CAD build for the part. Positions are in the model's coordinates, mm. A direction names the side the tool comes from. Coordinates: 2 decimals unless noted, no trailing zeros. Write each loop counter-clockwise with the first axis right and the second up, starting at its lowest first coordinate (ties: lowest second). Pieces come first, ordered by that corner, then holes. Notation, with made-up numbers: (65.25, 77) -> (98.25, 77) arc R28 cw to (98.25, 103) -> close; hole circle Ø3 at (31, -33). An arc over 180 degrees is marked (long way). Answer as CSV lines item,"result". Start each with the question number.
```python
from build123d import *

# Parameters (mm, degrees)
SKETCH1_R           = 12.5
BOSS_EXTRUDE1_DEPTH = 125
CUT_EXTRUDE1_START  = -20
CUT_EXTRUDE1_DEPTH  = 20
CHAMFER1_SIZE       = 2


with BuildPart() as part:
    # Sketch1 → Boss-Extrude1 (new body)
    with BuildSketch(Plane.XY):
        Circle(SKETCH1_R)
    extrude(amount=BOSS_EXTRUDE1_DEPTH)

    # Sketch2 → Cut-Extrude1 (cut)
    with BuildSketch(Plane.XY.offset(125).offset(CUT_EXTRUDE1_START)):
        with BuildLine():
            Line((-9.604686356, 8), (9.604686356, 8))
            ThreePointArc((9.604686356, 8), (0, 12.5), (-9.604686356, 8))
        make_face()
    extrude(amount=CUT_EXTRUDE1_DEPTH, mode=Mode.SUBTRACT)

    # Chamfer1
    chamfer1_edges = [part.edges().sort_by_distance(p)[0] for p in [
        (-12.5, 0, 0),
    ]]
    chamfer(chamfer1_edges, length=CHAMFER1_SIZE)


solid = part.part
```
1. Wall check: line 1 (X direction, y = 8, z = 46.5); line 2 (X direction, y = -9, z = 13); line 3 (Y direction, x = -7.25, z = 65.5). Give the ranges that are in metal, low to high.
2. Flat gauge pins, fed straight in: P1, Ø6, axis at y = -4.5, z = 97.5, coming from the +X side; P2, Ø3.5, axis at x = 3, y = 10, coming from the +Z side; P3, Ø1.5, axis at y = -1, z = 18, coming from the +X side; P4, Ø2, axis at x = -0.5, z = 27.5, coming from the -Y side. Where does each tip first touch, or does it go through?
3. Cut at A-A (x = 0). Give the cut face in (y, z), then the cut area to 3 significant figures.
4. Cut at B-B (z = 60.5). Give the cut face in (x, y).
5. Tool access for faces 1 (the face through (-2.71, -12.203, 62.639)), 2 (the face through (0, 10, 105)): list every direction of +Z, -Z, +X, -X, +Y, -Y with a clear straight run to the whole face (end or side of a thin tool).
Geometry check:
1,line 1,"-9.6 to 9.6"
1,line 2,"-8.67 to 8.67"
1,line 3,"-10.18 to 10.18"
2,P1,"x = 12.41"
2,P2,"z = 105"
2,P3,"x = 12.5"
2,P4,"y = -12.5"
3,outline,"(-12.5, 2) -> (-10.5, 0) -> (10.5, 0) -> (12.5, 2) -> (12.5, 105) -> (8, 105) -> (8, 125) -> (-12.5, 125) -> close"
3,area,"3,030 mm²"
4,outline,"circle Ø25 at (0, 0)"
5,face 1,"+Z, -Z"
5,face 2,"+Z, +X, -X, +Y"
